from build123d import *

# Parameters (mm, degrees)
F0_W     = 158.5
F0_H     = 56
F0_H_2   = 3.5
F0_W_2   = 3
F0_W_3   = 3.5
F1_DEPTH = 2
F2_D     = 3.5
F3_W     = 145
F3_H     = 63
F4_DEPTH = 4
F5_W     = 2
F5_H     = 22
F6_DEPTH = 8
F7_W     = 133
F7_H     = 55
F8_DEPTH = 6


with BuildPart() as f1:
    # F0 (on Front) → F1 (new body)
    with BuildSketch(Plane.XZ):
        with Locations((7.3379711658, -9.6212180674)):
            Rectangle(F0_W, F0_H)
        with Locations((7.3379711658, 20.1287819326)):
            Rectangle(F0_W, F0_H_2)
        with Locations((-73.4120288342, -9.6212180674)):
            Rectangle(F0_W_2, F0_H)
        with Locations((-73.4120288342, 20.1287819326)):
            Rectangle(F0_W_2, F0_H_2)
        with Locations((-73.4120288342, -39.3712180674)):
            Rectangle(F0_W_2, F0_H_2)
        with Locations((7.3379711658, -39.3712180674)):
            Rectangle(F0_W, F0_H_2)
        with Locations((88.3379711658, 20.1287819326)):
            Rectangle(F0_W_3, F0_H_2)
        with Locations((88.3379711658, -9.6212180674)):
            Rectangle(F0_W_3, F0_H)
        with Locations((88.3379711658, -39.3712180674)):
            Rectangle(F0_W_3, F0_H_2)
    extrude(amount=F1_DEPTH)

    # F2 (through all)
    with Locations(Plane(origin=(0, 0, 0), x_dir=(1, 0, 0), z_dir=(0, 1, 0))):
        with Locations((-71.9120288342, -18.3787819326), (86.5879711658, -18.3787819326), (86.5879711658, 37.6212180674), (-71.9120288342, 37.6212180674)):
            Hole(F2_D / 2)

    # F3 (on face) → F4 (join)
    with BuildSketch(Plane.XZ.offset(2)):
        with Locations((6.5879711658, -9.6212180674)):
            Rectangle(F3_W, F3_H)
    extrude(amount=F4_DEPTH)

    # F5 (on face) → F6 (join)
    with BuildSketch(Plane.YZ.offset(90.0879711658)):
        with Locations((-1, -7.1212180674)):
            Rectangle(F5_W, F5_H)
    extrude(amount=F6_DEPTH)

    # F7 (on face) → F8 (join)
    with BuildSketch(Plane.XZ.offset(6)):
        with Locations((6.5879711658, -8.6212180674)):
            Rectangle(F7_W, F7_H)
    extrude(amount=F8_DEPTH)


solid = f1.part
Here's how the part is built. I have some questions about the finished solid (model axes, mm). A direction names the side the tool comes from. Coordinates: 2 decimals unless noted, no trailing zeros. Order: outer loops, then holes, each group sorted by start corner. A loop starts at its lowest first (then second) coordinate and runs counter-clockwise, first axis right, second up. Notation, with made-up numbers: (41, 63) -> (89, 63) arc R35 cw to (89, 100) -> close; hole circle Ø8 at (18, 7). An arc over 180 degrees is marked (long way). Answer in a Markdown table with one row per item.
(1) On a 3-axis mill with a long thin cutter (end or side, diameter ignored), from which of +Z, -Z, +X, -X, +Y, -Y can I reach the whole of each face in a straight line? I mean faces 1 (the face through (73.088, -9, -9)), 2 (the face through (-70, -2, -9)), 3 (the face through (6, -9, 18.879)). Say none if no direction works.
Answer key:
| item | result |
|---|---|
| face 1 | +Z, -Z, +X, -Y |
| face 2 | +Z, -Z, -X, -Y |
| face 3 | +Z, +X, -X, -Y |
(2) I want a section at B-B on x = 32.5. List the corners of the cut face in (y, z) for me, then the cut area to 3 significant figures.
Answer key:
| item | result |
|---|---|
| outline | (-12, -36.12) -> (-6, -36.12) -> (-6, -41.12) -> (0, -41.12) -> (0, 21.88) -> (-6, 21.88) -> (-6, 18.88) -> (-12, 18.88) -> close |
| area | 708 mm^2 |
(3) Will these pins go through, and if not, where does the flat tip stop? pin 1 Ø9.5 at (x, z) = (87, -24) entering from -Y; pin 2 Ø1.5 at (y, z) = (-6.5, -12) entering from +X; pin 3 Ø4 at (y, z) = (-8.5, -28) entering from +X; pin 4 Ø3 at (x, z) = (-71.91, 18.38) entering from -Y.
Answer key:
| item | result |
|---|---|
| pin 1 | y = -2 |
| pin 2 | x = 79.09 |
| pin 3 | x = 73.09 |
| pin 4 | through |
(4) I want a section at A-A on z = -20. List the corners of the cut face in (x, y) for me, then the cut area to 3 significant figures.
Answer key:
| item | result |
|---|---|
| outline | (-74.91, -2) -> (-65.91, -2) -> (-65.91, -6) -> (-59.91, -6) -> (-59.91, -12) -> (73.09, -12) -> (73.09, -6) -> (79.09, -6) -> (79.09, -2) -> (90.09, -2) -> (90.09, 0) -> (-74.91, 0) -> close |
| area | 1,710 mm^2 |
(5) Please list where these lines run through material, in increasing order: probe 1 along X at (y, z) = (-8.25, -14); probe 2 along Z at (x, y) = (6, -8.5); probe 3 along X at (y, z) = (-0.75, 13).
Answer key:
| item | result |
|---|---|
| probe 1 | -59.91 to 73.09 |
| probe 2 | -36.12 to 18.88 |
| probe 3 | -74.91 to 90.09 |
(6) Thinking about a two-plate mould opening in X: for faces 4 (the face through (-59.912, -9, -9)), 5 (the face through (6, -9, -36.121)), 6 (the face through (84.92, -1.01, 17.85)), which applies, +X half, -X half, draft (parallel to the pull), parting line (faces both ways), or undercut?
Answer key:
| item | result |
|---|---|
| face 4 | -X half |
| face 5 | draft |
| face 6 | undercut |
(7) I want a section at C-C on y = -8. List the corners of the cut face in (x, z) for me.
Answer key:
| item | result |
|---|---|
| outline | (-59.91, -36.12) -> (73.09, -36.12) -> (73.09, 18.88) -> (-59.91, 18.88) -> close |
(8) I want a section at D-D on z = -11.5. List the corners of the cut face in (x, y) for me, then the cut area to 3 significant figures.
Answer key:
| item | result |
|---|---|
| outline | (-74.91, -2) -> (-65.91, -2) -> (-65.91, -6) -> (-59.91, -6) -> (-59.91, -12) -> (73.09, -12) -> (73.09, -6) -> (79.09, -6) -> (79.09, -2) -> (98.09, -2) -> (98.09, 0) -> (-74.91, 0) -> close |
| area | 1,720 mm^2 |
